Design review of the part built by this model. Coordinates are the model's own, in mm. A direction names the side the tool comes from. Coordinates: 2 decimals unless noted, no trailing zeros. Write each loop counter-clockwise with the first axis right and the second up, starting at its lowest first coordinate (ties: lowest second). Pieces come first, ordered by that corner, then holes. Notation, with made-up numbers: (-7, 74) - (2, 74) arc R21 cw to (2, 82) - close; hole circle Ø1 at (41.25, 84). An arc over 180 degrees is marked (long way). One line per item, written item: value.
from build123d import *

# Parameters (mm, degrees)
SKETCH_1_W          = 39
SKETCH_1_H          = 14
EXTRUDE_1_DEPTH     = 4
CUT_EXTRUDE_1_DEPTH = 2.5
SKETCH_3_R          = 1.125
CUT_EXTRUDE_2_DEPTH = 4
SKETCH_4_W          = 3.75
SKETCH_4_H          = 7
EXTRUDE_2_DEPTH     = 5
CUT_EXTRUDE_4_DEPTH = 14


with BuildPart() as part:
    # 스케치1 → 보스-돌출1 (new body)
    with BuildSketch(Plane(origin=(0, 0, 0), x_dir=(1, 0, 0), z_dir=(0, 1, 0))):
        Rectangle(SKETCH_1_W, SKETCH_1_H)
    extrude(amount=EXTRUDE_1_DEPTH)

    # 스케치2 → 컷-돌출1 (cut)
    with BuildSketch(Plane.XZ):
        Polygon((10.011473671, 0), (8.755736835, 2.175), (6.244263165, 2.175), (4.988526329, 0), (6.244263165, -2.175), (8.755736835, -2.175), align=None)
        Polygon((-4.988526329, 0), (-6.244263165, 2.175), (-8.755736835, 2.175), (-10.011473671, 0), (-8.755736835, -2.175), (-6.244263165, -2.175), align=None)
    extrude(amount=-CUT_EXTRUDE_1_DEPTH, mode=Mode.SUBTRACT)

    # 스케치3 → 컷-돌출2 (cut)
    with BuildSketch(Plane.XZ):
        with Locations((-7.5, 0)):
            Circle(SKETCH_3_R)
        with Locations((7.5, 0)):
            Circle(SKETCH_3_R)
    extrude(amount=-CUT_EXTRUDE_2_DEPTH, mode=Mode.SUBTRACT)

    # 스케치4 → 보스-돌출2 (add)
    with BuildSketch(Plane(origin=(0, 4, 0), x_dir=(1, 0, 0), z_dir=(0, 1, 0))):
        with Locations((-14.625, 0)):
            Rectangle(SKETCH_4_W, SKETCH_4_H)
        with Locations((14.625, 0)):
            Rectangle(SKETCH_4_W, SKETCH_4_H)
    extrude(amount=EXTRUDE_2_DEPTH)

    # 스케치5 → 컷-돌출4 (cut)
    with BuildSketch(Plane.XY.offset(7)):
        Polygon((-19.5, 1), (-19, 0), (-19.5, 0), align=None)
        Polygon((19.5, 1), (19.5, 0), (19, 0), align=None)
    extrude(amount=-CUT_EXTRUDE_4_DEPTH, mode=Mode.SUBTRACT)


solid = part.part
1. For faces 4 (the face through (-15, 6, -3.5)), 5 (the face through (-16.5, 6, 0)), 6 (the face through (12.75, 6, 0)), 7 (the face through (7, 1, -2.175)), list the 3-axis set-ups (+Z, -Z, +X, -X, +Y, -Y) from which the entire face can be reached by the end or side of a thin tool; tool diameter is ignored.
Answer block:
face 4: -Z, +X, -X, +Y
face 5: +Z, -Z, -X, +Y
face 6: +Z, -Z, +Y
face 7: -Y
2. Consider section C-C, the plane z = 0.75. Give the number of separate pieces and of enclosed holes in the cut face, then the cut area to 3 significant figures.
Answer block:
separate pieces: 3
enclosed holes: 0
area: 167 mm^2
3. Consider section D-D, the plane x = -1. Write out the cut boundary in (y, z).
Answer block:
outline: (0, -7) - (4, -7) - (4, 7) - (0, 7) - close
4. Mouldability with a two-part tool opening along Z and no side actions: class faces 1 (the face through (-9.375, 1.232, 1.103)), 2 (the face through (16.5, 6, 0)), 3 (the face through (15, 6, 3.5)) as released by +Z, released by -Z, zero draft, split by the parting line, or undercut.
Answer block:
face 1: undercut
face 2: zero draft
face 3: released by +Z
5. Consider section A-A, the plane y = 5.5. Write out the cut boundary in (x, z).
Answer block:
outline: (-16.5, -3.5) - (-12.75, -3.5) - (-12.75, 3.5) - (-16.5, 3.5) - close; (12.75, -3.5) - (16.5, -3.5) - (16.5, 3.5) - (12.75, 3.5) - close
6. Wall thickness on line 1 along Z through (x, y) = (7.5, 3.1) (3 decimals); line 2 along X through (y, z) = (8.5, -2.5); line 3 along Y through (x, z) = (-5.5, 1.5): over which ranges is each line inside the solid? List them lowest first.
Answer block:
line 1: z = -7 to -1.125, 1.125 to 7
line 2: x = -16.5 to -12.75, 12.75 to 16.5
line 3: y = 0 to 4
7. Consider section B-B, the plane x = -7.5. Write out the cut boundary in (y, z) (3 decimals), then the cut area to 4 significant figures.
Answer block:
outline: (0, -7) - (4, -7) - (4, -1.125) - (2.5, -1.125) - (2.5, -2.175) - (0, -2.175) - close; (0, 2.175) - (2.5, 2.175) - (2.5, 1.125) - (4, 1.125) - (4, 7) - (0, 7) - close
area: 41.75 mm^2
8. Insertion check: pin 1 Ø1.1 at (x, y) = (-14.5, 5.5) entering from +Z; pin 2 Ø1.3 at (x, z) = (-7.5, 0) entering from +Y; pin 3 Ø2.5 at (y, z) = (7, 0) entering from -X; pin 4 Ø2.5 at (y, z) = (7.5, 1.5) entering from +X. Each pin has a flat end and moves straight along its axis. Give the tip position at first contact, or say it passes through.
Answer block:
pin 1: stops at z = 3.5
pin 2: passes through
pin 3: stops at x = -16.5
pin 4: stops at x = 16.5
